Read the model definition and answer for the solid it produces. Units are mm, in the model's axes. A direction names the side the tool comes from. Give positions to 0.01 mm unless a question says otherwise; leave off trailing zeros. Put each result on its own line as item: value.
from build123d import *

# Parameters (mm, degrees)
RESSALTO_EXTRUS_O1_DEPTH = 5
ESBO_O3_R                = 2.25
CORTE_EXTRUS_O1_DEPTH    = 293.648462736


with BuildPart() as part:
    # Esboço1 → Ressalto-extrusão1 (new body)
    with BuildSketch(Plane.XY):
        with BuildLine():
            Line((-70, 50), (-70, 0))
            Line((-70, 0), (70, 0))
            Line((70, 0), (70, 50))
            Line((70, 50), (47.5, 50))
            Line((47.5, 50), (56.60599572, 100))
            add(Edge.make_bspline(
                [(56.60599572, 100), (58.822881578, 111.230467147), (70.624101453, 157.653217098), (70.983496175, 170.948411875), (70, 200)],
                knots=[0, 0, 0, 0, 0.304799144, 1, 1, 1, 1], degree=3))
            add(Edge.make_bspline(
                [(70, 200), (54.940172813, 213.077606657), (36.4, 208.4)],
                knots=[0, 0, 0, 1, 1, 1], degree=2))
            add(Edge.make_bspline(
                [(36.4, 208.4), (36.384425779, 208.408148411), (31.853718899, 218.695035342), (19.625229428, 225.496752597), (14.287120073, 225.126645694), (14, 225.2)],
                knots=[0, 0, 0, 0, 0.552885048, 0.635199122, 0.823140743, 0.823140743, 0.823140743, 0.823140743], degree=3))
            Line((14, 225.2), (14, 236.488415854))
            ThreePointArc((14, 236.488415854), (14.0946545, 236.599459291), (14.172142078, 236.723095026))
            add(Edge.make_bspline(
                [(14.172142078, 236.723095026), (16.438682622, 241.005058154), (19.848023934, 251.961326161), (20.98093901, 253.933353369), (21, 263)],
                knots=[0.009275677, 0.009275677, 0.009275677, 0.009275677, 0.377960332, 0.746644988, 0.746644988, 0.746644988, 0.746644988], degree=3))
            ThreePointArc((21, 263), (0, 284), (-21, 263))
            add(Edge.make_bspline(
                [(-14.172142078, 236.723095026), (-16.438682622, 241.005058154), (-19.848023934, 251.961326161), (-20.98093901, 253.933353369), (-21, 263)],
                knots=[0.009275677, 0.009275677, 0.009275677, 0.009275677, 0.377960332, 0.746644988, 0.746644988, 0.746644988, 0.746644988], degree=3))
            ThreePointArc((-14.172142078, 236.723095026), (-14.0946545, 236.599459291), (-14, 236.488415854))
            Line((-14, 236.488415854), (-14, 225.2))
            add(Edge.make_bspline(
                [(-36.4, 208.4), (-36.384425779, 208.408148411), (-31.853718899, 218.695035342), (-19.625229428, 225.496752597), (-14.287120073, 225.126645694), (-14, 225.2)],
                knots=[0, 0, 0, 0, 0.552885048, 0.635199122, 0.823140743, 0.823140743, 0.823140743, 0.823140743], degree=3))
            add(Edge.make_bspline(
                [(-70, 200), (-54.940172813, 213.077606657), (-36.4, 208.4)],
                knots=[0, 0, 0, 1, 1, 1], degree=2))
            add(Edge.make_bspline(
                [(-56.60599572, 100), (-58.822881578, 111.230467147), (-70.624101453, 157.653217098), (-70.983496175, 170.948411875), (-70, 200)],
                knots=[0, 0, 0, 0, 0.304799144, 1, 1, 1, 1], degree=3))
            Line((-56.60599572, 100), (-47.5, 50))
            Line((-47.5, 50), (-70, 50))
        make_face()
    extrude(amount=RESSALTO_EXTRUS_O1_DEPTH)

    # Esboço3 → Corte-extrusão1 (cut, through all)
    with BuildSketch(Plane.XY.offset(5)):
        with Locations((-56.3, 182.2)):
            Circle(ESBO_O3_R)
        with Locations(Location((56.3, 182.2, 0), (0, 0, 180))):
            Circle(ESBO_O3_R)
    extrude(amount=-CORTE_EXTRUS_O1_DEPTH, mode=Mode.SUBTRACT)


solid = part.part
(1) Section A-A on z = 1 is taken. Give the number of separate pieces and of enclosed holes in the cut face, and give its area (3 significant figures).
Result:
separate pieces: 1
enclosed holes: 2
area: 29,500 mm²
(2) Straight lines are drawn through the part: line 1 along X through (y, z) = (182.2, 1.05); line 2 along X through (y, z) = (184, 1.8); line 3 along Y through (x, z) = (46, 0.7). For each, find the intervals that lie inside material, in ascending order. Write a range as from..to.
Result:
line 1: x = -70.43..-58.55, -54.05..54.05, 58.55..70.43
line 2: x = -70.42..-57.65, -54.95..54.95, 57.65..70.42
line 3: y = 0..209.63
(3) For a pull along Y with two mould halves and no side action, classify faces 1 (the face through (-1, 0, 2)), 2 (the face through (70, 25, 2)), 3 (the face through (-52.117, 75.35, 2.465)) as +Y half, -Y half, draft (parallel to the pull), parting line (faces both ways), or undercut.
Result:
face 1: -Y half
face 2: draft
face 3: undercut
(4) Given pin 1 Ø2.5 at (y, z) = (32, 1.5) entering from +X; pin 2 Ø1.5 at (y, z) = (232, 3) entering from -X; pin 3 Ø2 at (x, z) = (39.5, 0.5) entering from +Y; pin 4 Ø2.5 at (x, y) = (-56.3, 182.2) entering from -Z, each flat-ended and moving along its own axis, determine where each tip first touches the part or whether it passes through.
Result:
pin 1: stops at x = 70
pin 2: stops at x = -14
pin 3: stops at y = 209.22
pin 4: passes through
(5) Which of the six approach directions +Z, -Z, +X, -X, +Y, -Y give full straight-line access (tool end or side, diameter ignored) to faces 4 (the face through (-70, 25, 2)), 5 (the face through (-59, 50, 2)), 6 (the face through (59, 50, 2)), 7 (the face through (0, 284, 2)), 8 (the face through (-1, 112, 5))?
Result:
face 4: +Z, -Z, -X, -Y
face 5: +Z, -Z, -X
face 6: +Z, -Z, +X
face 7: +Z, -Z, +Y
face 8: +Z, +X, -X, +Y, -Y
